Drawing for the job (mm, zero at the part's lowest x, y, z). A direction names the side the tool comes from. Give positions to 0.01 mm unless a question says otherwise; leave off trailing zeros. Write each loop counter-clockwise with the first axis right and the second up, starting at its lowest first coordinate (ties: lowest second). Pieces come first, ordered by that corner, then holes. Notation, with made-up numbers: M 41.5,38 L 93.5,38 A31 cw 93.5,77 Z; hole C 84.5,46.25 d7. An arc over 180 degrees is marked long. Use a Markdown table: item, result. Add a question column.
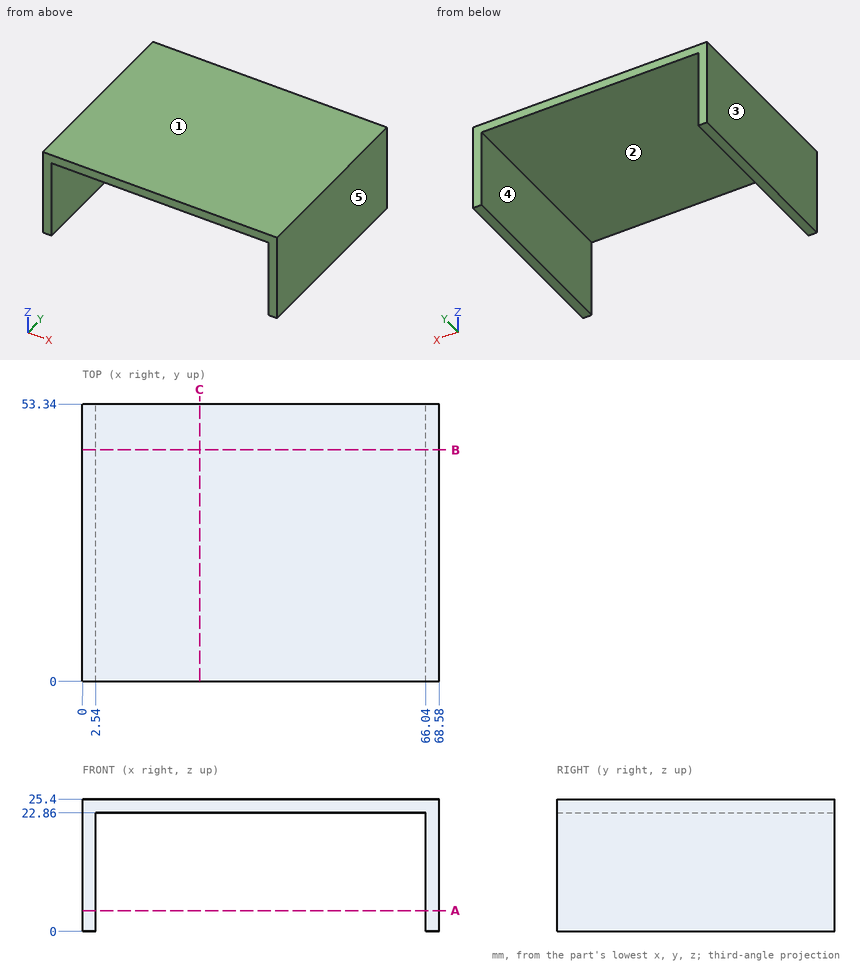
1. Drill centre lines: probe 1 along X at (y, z) = (13, 3); probe 2 along Z at (x, y) = (51, 25.5). Where is each one in solid material? Low to high. Write a range as [from, to].
2. Tool access for the marked faces 1 and 2: list every direction of +Z, -Z, +X, -X, +Y, -Y with a clear straight run to the whole face (end or side of a thin tool).
3. Cut at B-B (y = 44.5). Write the cut outline in (x, z), then the cut area to 3 significant figures.
4. Flat gauge pins, fed straight in: pin 1 (5 mm diameter, centred on x = 53.5, y = 42, fed in from -Z); pin 2 (1 mm diameter, centred on y = 6, z = 18.5, fed in from -X). Where does each tip first touch, or does it go through?
5. Cut at A-A (z = 4). Write the cut outline in (x, y), then the cut area to 3 significant figures.
6. Mould opens along X. For the marked faces 3, 4 and 5 say: released by +X, released by -X, zero draft, split by the parting line, or undercut.
7. Cut at C-C (x = 22.5). Write the cut outline in (y, z), then the cut area to 3 significant figures.
A:
| question | item | result |
|---|---|---|
| 1 | probe 1 | x = [0, 2.54], [66.04, 68.58] |
| 1 | probe 2 | z = [22.86, 25.4] |
| 2 | face 1 | +Z, +X, -X, +Y, -Y |
| 2 | face 2 | -Z, +Y, -Y |
| 3 | outline | M 0,0 L 2.54,0 L 2.54,22.86 L 66.04,22.86 L 66.04,0 L 68.58,0 L 68.58,25.4 L 0,25.4 Z |
| 3 | area | 290 mm² |
| 4 | pin 1 | stops at z = 22.86 |
| 4 | pin 2 | stops at x = 0 |
| 5 | outline | M 0,0 L 2.54,0 L 2.54,53.34 L 0,53.34 Z; M 66.04,0 L 68.58,0 L 68.58,53.34 L 66.04,53.34 Z |
| 5 | area | 271 mm² |
| 6 | face 3 | released by -X |
| 6 | face 4 | undercut |
| 6 | face 5 | released by +X |
| 7 | outline | M 0,22.86 L 53.34,22.86 L 53.34,25.4 L 0,25.4 Z |
| 7 | area | 135 mm² |
